Geometry check sheet. Reference: the model listing, model coordinates, mm. A direction names the side the tool comes from. Round coordinates to 2 decimals unless told otherwise and drop trailing zeros. Write each loop counter-clockwise with the first axis right and the second up, starting at its lowest first coordinate (ties: lowest second). Pieces come first, ordered by that corner, then holes. Notation, with made-up numbers: M -39,53.25 L -26,53.25 A35 cw -26,89.25 Z; hole C 37,-4.75 d1. An arc over 180 degrees is marked long. Use a Markdown table: item, result.
```python
from build123d import *

# Parameters (mm, degrees)
F1_DEPTH = 50.8
F3_DEPTH = 518.2199364311
F5_DEPTH = 25.4


with BuildPart() as f1:
    # F0 (on Top) → F1 (new body)
    with BuildSketch(Plane.XY):
        Polygon((-256.483467652, 156.1972611251), (-518.2189364311, 0), (5.2520011271, 0), align=None)
    extrude(amount=F1_DEPTH)

    # F2 (on Right) → F3 (cut, through all)
    with BuildSketch(Plane.YZ):
        Polygon((6.7202083301, 38.1), (0, 30.48), (0, 20.32), (6.7202083301, 12.7), align=None)
    extrude(amount=-F3_DEPTH, mode=Mode.SUBTRACT)

    # F4 (on face) → F5 (join)
    with BuildSketch(Plane.XY.offset(50.8)):
        with BuildLine():
            Line((-363.5565638542, 66.0699382424), (-363.5565638542, 15.4361305758))
            Line((-363.5565638542, 15.4361305758), (-348.9585369825, 15.4361305758))
            Line((-348.9585369825, 15.4361305758), (-348.9585369825, 66.7609721422))
            add(Edge.make_bspline(
                [(-348.9585369825, 66.7609721422), (-349.1962850094, 72.1294507384), (-349.340803371, 85.5928406176), (-287.6615089898, 84.1058113884), (-262.8928370601, 81.391743052), (-262.399105211, 55.5299626512), (-262.4850422144, 40.7699868083)],
                knots=[0, 0, 0, 0, 0.1668742466, 0.5097494757, 0.7240103804, 1, 1, 1, 1], degree=3))
            Line((-262.4850422144, 40.7699868083), (-262.4850422144, 23.5870201141))
            Line((-262.4850422144, 23.5870201141), (-246.4926242828, 23.5870201141))
            Line((-246.4926242828, 23.5870201141), (-246.4926242828, 31.2213213871))
            Line((-246.4926242828, 31.2213213871), (-143.9413215727, 69.1381444045))
            Line((-143.9413215727, 69.1381444045), (-143.9413215727, 89.0348888997))
            Line((-143.9413215727, 89.0348888997), (-246.4926242828, 46.603564173))
            add(Edge.make_bspline(
                [(-363.5565638542, 66.0699382424), (-363.2831573486, 71.5237334371), (-365.6765544545, 78.9120083056), (-355.040460294, 96.3197217064), (-331.9011142788, 100.4510749559), (-301.9417077036, 98.9408625209), (-274.3425806674, 99.936876108), (-247.8596834541, 92.3872071167), (-248.6338026523, 64.1174365029), (-247.7710895443, 55.5507833564), (-246.4926242828, 46.603564173)],
                knots=[0, 0, 0, 0, 0.0967978336, 0.2071312198, 0.3339171066, 0.4812298803, 0.6246455368, 0.7535419216, 0.8817715915, 1, 1, 1, 1], degree=3))
        make_face()
        Polygon((-363.5565638542, 15.4361305758), (-363.5565638542, 0), (-141.8597176671, 0), (-141.8597176671, 15.4361305758), (-348.9585369825, 15.4361305758), align=None)
    extrude(amount=F5_DEPTH)


solid = f1.part
```
Item 1: Access from +Z, -Z, +X, -X, +Y, -Y to the whole of each face (thin tool, end or side, straight path). Record for faces 1 (the face through (-143.941, 79, 63)), 2 (the face through (-194.499, 68.116, 63.322)), 3 (the face through (-348.959, 41, 63)).
Outcome:
| item | result |
|---|---|
| face 1 | +Z, +X, +Y |
| face 2 | +Z, +Y |
| face 3 | +Z |
Item 2: Cross-section at B-B, the plane y = 135. Record the cut outline in (x, z), and give its area (3 significant figures).
Outcome:
| item | result |
|---|---|
| outline | M -292,0 L -220.96,0 L -220.96,50.8 L -292,50.8 Z |
| area | 3,610 mm2 |
Item 3: Material ranges on line 1 along Z through (x, y) = (-181.5, 25); line 2 along Y through (x, z) = (-185, 33.5); line 3 along X through (y, z) = (63, 21), recorded low to high. Write a range as from..to.
Outcome:
| item | result |
|---|---|
| line 1 | z = 0..50.8 |
| line 2 | y = 0..2.66, 6.72..113.54 |
| line 3 | x = -412.65..-100.32 |
Item 4: Cross-section at A-A, the plane x = -377. Record the cut outline in (y, z).
Outcome:
| item | result |
|---|---|
| outline | M 0,0 L 84.28,0 L 84.28,50.8 L 0,50.8 L 0,30.48 L 6.72,38.1 L 6.72,12.7 L 0,20.32 Z |
Item 5: Cross-section at C-C, the plane x = -83. Record the cut outline in (y, z).
Outcome:
| item | result |
|---|---|
| outline | M 0,0 L 52.67,0 L 52.67,50.8 L 0,50.8 L 0,30.48 L 6.72,38.1 L 6.72,12.7 L 0,20.32 Z |
Item 6: Cross-section at D-D, the plane y = 114. Record the cut outline in (x, z), and give its area (3 significant figures).
Outcome:
| item | result |
|---|---|
| outline | M -327.19,0 L -185.77,0 L -185.77,50.8 L -327.19,50.8 Z |
| area | 7,180 mm2 |
Item 7: Go/stop test with flat-tipped pins: pin 1 (10 mm diameter, centred on x = -342, z = 26, fed in from +Y); pin 2 (20.5 mm diameter, centred on y = 24, z = 65, fed in from -X); pin 3 (2.5 mm diameter, centred on y = 26.5, z = 68, fed in from +X). Record where each tip stops, or that it passes through.
Outcome:
| item | result |
|---|---|
| pin 1 | stops at y = 108.15 |
| pin 2 | stops at x = -363.56 |
| pin 3 | stops at x = -246.49 |
Item 8: Mould release check, pull along Z, two halves, no side actions. Record for faces 4 (the face through (-253, 6.72, 25)), 5 (the face through (-318, 107, 50.8)), 6 (the face through (-385.52, 79.19, 25.04)): +Z half, -Z half, draft (parallel to the pull), parting line (faces both ways), or undercut.
Outcome:
| item | result |
|---|---|
| face 4 | undercut |
| face 5 | +Z half |
| face 6 | draft |
